Source: CAD feature listing. Evaluate the final solid. Frame: model axes, mm. Face numbers are marked on the shaded views. Coordinates: 2 decimals unless noted, no trailing zeros. Write each loop counter-clockwise with the first axis right and the second up, starting at its lowest first coordinate (ties: lowest second). Pieces come first, ordered by that corner, then holes. Notation, with made-up numbers: (26.25, -14.5) - (78.25, -14.5) arc R12 cw to (78.25, -10.5) - close; hole circle Ø10 at (74, -24.75). An arc over 180 degrees is marked (long way). One line per item, written item: value.
from build123d import *

# Parameters (mm, degrees)
SKETCH_1_W          = 40
SKETCH_1_H          = 40
EXTRUDE_2_DEPTH     = 46.5
SKETCH_3_W          = 38.5
SKETCH_3_H          = 20
EXTRUDE_3_DEPTH     = 2.75
SKETCH_4_W          = 38.5
SKETCH_4_H          = 20
EXTRUDE_4_DEPTH     = 2.75
CUT_EXTRUDE_1_DEPTH = 38
SKETCH_6_R          = 7.5
EXTRUDE_5_DEPTH     = 48.5
EXTRUDE_START       = -50.5
SKETCH_7_R          = 7.5
EXTRUDE_6_DEPTH     = 50.5
FILLET_1_R          = 10
SKETCH_8_R          = 4
CUT_EXTRUDE_2_DEPTH = 50.5
SKETCH_9_R          = 6
EXTRUDE_7_DEPTH     = 6
SKETCH_10_R         = 4
EXTRUDE_9_DEPTH     = 20
FILLET_3_R          = 6


# Some blends are built 0.0001 mm under size
with BuildPart() as part:
    # 草图1 → 凸台-拉伸2 (new body)
    with BuildSketch(Plane(origin=(0, 0, 0), x_dir=(0, 0, -1), z_dir=(1, 0, 0))):
        with Locations((1.325599553, 10.998115505)):
            Rectangle(SKETCH_1_W, SKETCH_1_H)
    extrude(amount=EXTRUDE_2_DEPTH)

    # 草图3 → 凸台-拉伸3 (add)
    with BuildSketch(Plane(origin=(46.5, 0, 0), x_dir=(0, 0, -1), z_dir=(1, 0, 0))):
        with Locations((-37.924400447, 0.998115505)):
            Rectangle(SKETCH_3_W, SKETCH_3_H)
    extrude(amount=-EXTRUDE_3_DEPTH)

    # 草图4 → 凸台-拉伸4 (add)
    with BuildSketch(Plane.ZY):
        with Locations((37.924400447, 0.998115505)):
            Rectangle(SKETCH_4_W, SKETCH_4_H)
    extrude(amount=-EXTRUDE_4_DEPTH)

    # 草图5 → 切除-拉伸1 (cut)
    with BuildSketch(Plane.XY.offset(18.674400447)):
        Polygon((2.75, 10.998115505), (2.75, 30.998115505), (43.75, 30.998115505), (43.75, 10.998115505), (43.75, -9.001884495), (2.75, -9.001884495), align=None)
    extrude(amount=-CUT_EXTRUDE_1_DEPTH, mode=Mode.SUBTRACT)

    # 草图6 → 凸台-拉伸5 (add)
    with BuildSketch(Plane.ZY):
        with Locations((-1.325599553, 20.998115505)):
            Circle(SKETCH_6_R)
    extrude(amount=-EXTRUDE_5_DEPTH)

    # 草图7 → 凸台-拉伸6 (add)
    with BuildSketch(Plane(origin=(48.5, 0, 0), x_dir=(0, 0, -1), z_dir=(1, 0, 0)).offset(EXTRUDE_START)):
        with Locations(Location((1.325599553, 20.998115505, 0), (0, 0, 180))):
            Circle(SKETCH_7_R)
    extrude(amount=EXTRUDE_6_DEPTH)

    # 圆角1
    # the kernel refuses this fillet: 10 mm, written as the material it takes off along each edge
    with BuildSketch(Plane(origin=(48.5, 20.998115505, -1.325599553), x_dir=(0, 0, 1), z_dir=(0, -1, 0))) as fillet_1_piece_1:
        with BuildLine():
            CenterArc((1.5, 10), FILLET_1_R, 270, 36.869897646)
            Line((1.5, 0), (1.5, -0.2))
            Line((1.5, -0.2), (7.5, -0.2))
            Line((7.5, -0.2), (7.7, 0))
            ThreePointArc((7.7, 0), (7.7, 1), (7.62, 1.84))
            Line((7.62, 1.84), (7.5, 2))
        make_face()
    revolve(axis=Axis((48.5, 20.998115505, -1.325599553), (-1, 0, 0)), mode=Mode.SUBTRACT)
    with BuildSketch(Plane(origin=(-2, 20.998115505, -1.325599553), x_dir=(0, 0, 1), z_dir=(0, 1, 0))) as fillet_1_piece_2:
        with BuildLine():
            CenterArc((1.5, 10), FILLET_1_R, 270, 36.869897646)
            Line((1.5, 0), (1.5, -0.2))
            Line((1.5, -0.2), (7.5, -0.2))
            Line((7.5, -0.2), (7.7, 0))
            ThreePointArc((7.7, 0), (7.7, 1), (7.62, 1.84))
            Line((7.62, 1.84), (7.5, 2))
        make_face()
    revolve(axis=Axis((-2, 20.998115505, -1.325599553), (1, 0, 0)), mode=Mode.SUBTRACT)

    # 草图8 → 切除-拉伸2 (cut)
    with BuildSketch(Plane(origin=(46.5, 0, 0), x_dir=(0, 0, -1), z_dir=(1, 0, 0))):
        with Locations((-41.863292437, 0.998115505)):
            Circle(SKETCH_8_R)
        with Locations((-29.525991128, 0.998115505)):
            Circle(SKETCH_8_R)
    extrude(amount=-CUT_EXTRUDE_2_DEPTH, mode=Mode.SUBTRACT)

    # 草图9 → 凸台-拉伸7 (add)
    with BuildSketch(Plane(origin=(0, 0, -21.325599553), x_dir=(-1, 0, 0), z_dir=(0, 0, -1))):
        with Locations((-23.25, 20.998115505)):
            Circle(SKETCH_9_R)
    extrude(amount=EXTRUDE_7_DEPTH)

    # 草图10 → 凸台-拉伸9 (add)
    with BuildSketch(Plane(origin=(0, 0, -27.325599553), x_dir=(-1, 0, 0), z_dir=(0, 0, -1))):
        with Locations((-23.25, 20.998115505)):
            Circle(SKETCH_10_R)
    extrude(amount=-EXTRUDE_9_DEPTH)

    # 圆角3
    fillet_3_edges = [part.edges().sort_by_distance(p)[0] for p in [
        (29.25, 20.998115505, -27.325599553),
    ]]
    fillet(fillet_3_edges, radius=FILLET_3_R - 0.0001)  # a hair under: the kernel refuses the full size


solid = part.part
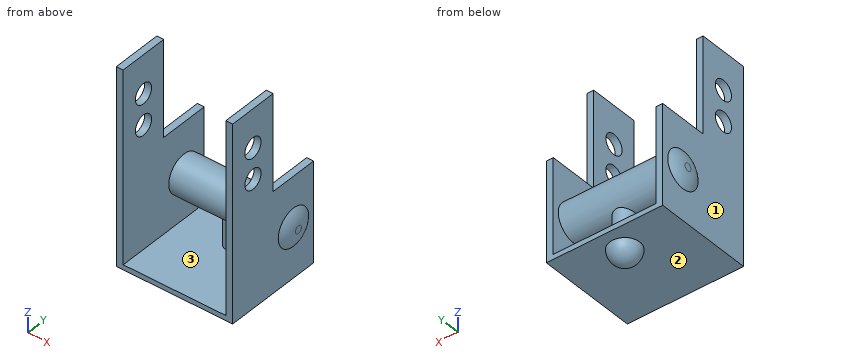
1) Section query C-C on z = 44.5. Output: boundary loops of the cut face in (x, y).
Values found:
outline: (0, -9) - (2.75, -9) - (2.75, -2.01) - (0, -2.01) - close; (0, 4.01) - (2.75, 4.01) - (2.75, 11) - (0, 11) - close; (43.75, -9) - (46.5, -9) - (46.5, -2.01) - (43.75, -2.01) - close; (43.75, 4.01) - (46.5, 4.01) - (46.5, 11) - (43.75, 11) - close
2) Section query B-B on x = 41.5. Output: boundary loops of the cut face in (y, z).
Values found:
outline: (-9, -21.33) - (31, -21.33) - (31, -19.33) - (-9, -19.33) - close; circle Ø15 at (21, -1.33)
3) Section query A-A on z = 35. Output: boundary loops of the cut face in (x, y), then the cut area to 3 significant figures.
Values found:
outline: (0, -9) - (2.75, -9) - (2.75, 11) - (0, 11) - close; (43.75, -9) - (46.5, -9) - (46.5, 11) - (43.75, 11) - close
area: 110 mm2
4) Contact query for flat-ended pins moving along their axis: P1, Ø0.8, axis at x = 1.5, z = 37.5, coming from the +Y side; P2, Ø2, axis at x = 45.5, y = 24, coming from the +Z side; P3, Ø1, axis at x = 24.5, z = 4, coming from the +Y side; P4, Ø20, axis at y = 16.5, z = -1, coming from the +X side. Output: stop coordinate, or through.
Values found:
P1: y = 11
P2: z = 18.67
P3: y = 26.74
P4: x = 48.5
5) Material intervals for line 1 (X direction, y = 8, z = 17); line 2 (Z direction, x = 34.5, y = 21); line 3 (Z direction, x = 1.5, y = 22), sorted ascending.
Values found:
line 1: 0 to 2.75, 43.75 to 46.5
line 2: -21.33 to -19.33, -8.83 to 6.17
line 3: -21.33 to 18.67
6) Draft query along Z for the marked faces 1, 2 and 3. Return one class per face: released by +Z, released by -Z, zero draft, split by the parting line, or undercut.
Values found:
face 1: zero draft
face 2: released by -Z
face 3: undercut
7) Section query D-D on y = 6. Output: boundary loops of the cut face in (x, z), then the cut area to 3 significant figures.
Values found:
outline: (0, -21.33) - (46.5, -21.33) - (46.5, 57.17) - (43.75, 57.17) - (43.75, -19.33) - (2.75, -19.33) - (2.75, 57.17) - (0, 57.17) - close
area: 514 mm2
